```python
from build123d import *

# Parameters (mm, degrees)
F0_R     = 50
F1_DEPTH = 5
F3_R     = 2
F2_R     = 45
F4_DEPTH = 15
F5_T     = 2.5
F6_R     = 5


# Not quite as in the source:
# - a shell that OpenCascade refuses in one call is made with other operations: the cavity is built on its own and cut out


with BuildPart() as f1:
    # F0 (on Front) → F1 (new body)
    with BuildSketch(Plane.XZ):
        Circle(F0_R)
    extrude(amount=F1_DEPTH)

    # F3
    f3_edges = [f1.edges().sort_by_distance(p)[0] for p in [
        (-50, -5, 0),
        (-50, 0, 0),
    ]]
    fillet(f3_edges, radius=F3_R)

    # F2 (on Front) → F4 (join)
    with BuildSketch(Plane.XZ):
        Circle(F2_R)
    extrude(amount=F4_DEPTH)

    # F5: shell of thickness 2.5, made by hand


with BuildPart() as f5_core1:
    # F5_t2: copy of F1
    add(f1.part)

    # the walls: a layer under each face that stays
    f5_faces = [f5_core1.faces().sort_by_distance(p)[0] for p in [
        (-50, -2.5, 0),
        (0, 0, 0),
        (-32, -5, -32),
        (-45, -10, 0),
    ]]
    thicken(f5_faces, amount=-F5_T, mode=Mode.SUBTRACT)

    # F5_s3 → F5_t4 (revolve, cut)
    with BuildSketch(Plane.XY):
        Polygon((45.025, -5.025), (45, -2.5), (42.5, -2.5), (42.5, -5), align=None)
    revolve(axis=Axis((0, -5, 0), (0, 1, 0)), mode=Mode.SUBTRACT)


with BuildPart() as f1_1:
    add(f1.part)

    # what is left inside the walls is the cavity
    f5_cavity = [f5_core1.part.solids().sort_by_distance(p)[0] for p in [
        (0, -2.525, -14.166667),
    ]]
    add(f5_cavity, mode=Mode.SUBTRACT)

    # F6
    f6_edges = [f1_1.edges().sort_by_distance(p)[0] for p in [
        (42.5, -8.75, 0),
        (-42.5, -2.5, 0),
    ]]
    fillet(f6_edges, radius=F6_R)


solid = f1_1.part
```
The model under review builds one solid part; all positions refer to its coordinate system, in mm. A direction names the side the tool comes from. Coordinates: 2 decimals unless noted, no trailing zeros. Write each loop counter-clockwise with the first axis right and the second up, starting at its lowest first coordinate (ties: lowest second). Pieces come first, ordered by that corner, then holes. Notation, with made-up numbers: (28.25, 58.5) -> (68.25, 58.5) arc R23 ccw to (68.25, 84.5) -> close; hole circle Ø4 at (19, 28.25). An arc over 180 degrees is marked (long way). One line per item, written item: value. Start each with the question number.
Q1. To check wall thickness, follow probe 1 along X at (y, z) = (-9.25, 0); probe 2 along X at (y, z) = (-13.5, -18). State the ranges of each line that lie inside material, in increasing order.
Q2. Clearance check with flat-ended pins moving along their axes: P1, Ø6, axis at y = -3.5, z = -30, coming from the +X side; P2, Ø6, axis at x = -21, y = -12, coming from the +Z side; P3, Ø4, axis at x = 21.5, y = -4.5, coming from the +Z side. State where each tip first meets the part, or that it passes through.
Q3. Add section C-C, the plane z = 0. Give the boundary of the cut face in (x, y), then the cut area to 3 significant figures.
Q4. Add section B-B, the plane y = -10.75. Give the boundary of the cut face in (x, z), then the cut area to 3 significant figures.
Q5. For faces 4 (the face through (-26.9, -15, -33.1)), 5 (the face through (14, -5, 43)), list the 3-axis set-ups (+Z, -Z, +X, -X, +Y, -Y) from which the entire face can be reached by the end or side of a thin tool; tool diameter is ignored.
Q6. Add section A-A, the plane x = 0. Give the boundary of the cut face in (y, z), then the cut area to 3 significant figures.
Q7. The part is to be moulded in two halves that separate along Z. For faces 1 (the face through (20.765, -9.93, -39.923)), 2 (the face through (-33.727, -11.198, -25.861)), 3 (the face through (-1, 0, 1)), say which applies: +Z half, -Z half, draft (parallel to the pull), parting line (faces both ways), or undercut.
Response:
1. probe 1: -45 to -42.5, 42.5 to 45
1. probe 2: -41.24 to -38.5, 38.5 to 41.24
2. P1: x = 42.06
2. P2: z = 41.24
2. P3: z = 45.86
3. outline: (-50, -3) arc R2 ccw to (-48, -5) -> (-45, -5) -> (-45, -15) -> (-42.5, -15) -> (-42.5, -7.5) arc R5 cw to (-37.5, -2.5) -> (37.5, -2.5) arc R5 cw to (42.5, -7.5) -> (42.5, -15) -> (45, -15) -> (45, -5) -> (48, -5) arc R2 ccw to (50, -3) -> (50, -2) arc R2 ccw to (48, 0) -> (-48, 0) arc R2 ccw to (-50, -2) -> close
3. area: 345 mm²
4. outline: circle Ø90 at (0, 0); hole circle Ø85 at (0, 0)
4. area: 687 mm²
5. face 4: +Z, -Z, +X, -X, -Y
5. face 5: -Y
6. outline: (-15, -45) -> (-5, -45) -> (-5, -48) arc R2 ccw to (-3, -50) -> (-2, -50) arc R2 ccw to (0, -48) -> (0, 48) arc R2 ccw to (-2, 50) -> (-3, 50) arc R2 ccw to (-5, 48) -> (-5, 45) -> (-15, 45) -> (-15, 42.5) -> (-7.5, 42.5) arc R5 cw to (-2.5, 37.5) -> (-2.5, -37.5) arc R5 cw to (-7.5, -42.5) -> (-15, -42.5) -> close
6. area: 345 mm²
7. face 1: parting line
7. face 2: undercut
7. face 3: draft
